```python
from build123d import *

# Parameters (mm, degrees)
SKETCH2_R                 = 3.2
FRONT_MOUNTING_DEPTH      = 10.65
FRONT_MOUNTING_DEPTH_BACK = 10.65


with BuildPart() as part:
    # Sketch1 → Body (revolve)
    with BuildSketch(Plane(origin=(0, 0, 0), x_dir=(0, 0, -1), z_dir=(1, 0, 0))):
        Polygon((51.45, 9.65), (50.2, 8.4), (48.95, 9.65), (-31, 9.65), (-31, 0), (67.4, 0), (67.4, 9.65), (57.7, 9.65), align=None)
    revolve(axis=Axis((0, 0, -67.4), (0, 0, 1)))

    # Sketch2 → Front-Mounting (cut, two sides)
    with BuildSketch(Plane(origin=(0, 0, 0), x_dir=(0, 0, -1), z_dir=(1, 0, 0))) as front_mounting_sk:
        with Locations((57.7, 0)):
            Circle(SKETCH2_R)
    extrude(amount=FRONT_MOUNTING_DEPTH, mode=Mode.SUBTRACT)
    extrude(front_mounting_sk.sketch, amount=-FRONT_MOUNTING_DEPTH_BACK, mode=Mode.SUBTRACT)


solid = part.part
```
The listing builds one solid part. Answer for the finished solid, in the listing's coordinates (mm). A direction names the side the tool comes from. Round coordinates to 2 decimals unless told otherwise and drop trailing zeros. Loops run counter-clockwise (first coordinate to the right, second up) from the corner with the lowest first, then second, coordinate; pieces in that order, holes last.
1) A cutting plane is placed at C-C on z = -53. Determine the outline of the cut face in (x, y), plus the area to 3 significant figures.
Outcome:
outline: circle Ø19.3 at (0, 0)
area: 293 mm2
2) Given P1, Ø1.5, axis at x = 5, z = -3, coming from the -Y side; P2, Ø6, axis at x = -6, z = -6.5, coming from the +Y side; P3, Ø6, axis at y = 0, z = -57.7, coming from the -X side; P4, Ø6, axis at y = -4, z = -50.5, coming from the +X side, each flat-ended and moving along its own axis, determine where each tip first touches the part or whether it passes through.
Outcome:
P1: stops at y = -8.66
P2: stops at y = 9.17
P3: passes through
P4: stops at x = 9.58
3) For a pull along Z with two mould halves and no side action, classify faces 3 (the face through (-2.899, 9.204, -8.415)), 4 (the face through (0, 0, 31)), 5 (the face through (0.1, 0.1, -54.5)) as released by +Z, released by -Z, zero draft, split by the parting line, or undercut.
Outcome:
face 3: zero draft
face 4: released by +Z
face 5: undercut
4) For faces 1 (the face through (0, 0, -67.4)), 2 (the face through (-7, 5, -50)), determine the directions among +Z, -Z, +X, -X, +Y, -Y from which every point of the face is accessible in a straight line to the end or side of a thin tool.
Outcome:
face 1: -Z, +X, -X, +Y, -Y
face 2: none
5) Consider line 1 (Z direction, x = -1, y = 0); line 2 (Z direction, x = -0.5, y = 0.75); line 3 (Y direction, x = 5.75, z = -57.5). Determine where each line is inside the solid, lowest interval first.
Outcome:
line 1: z = -67.4 to -60.9, -54.5 to 31
line 2: z = -67.4 to -60.81, -54.59 to 31
line 3: y = -7.75 to -3.19, 3.19 to 7.75
6) A cutting plane is placed at A-A on x = 0. Determine the outline of the cut face in (y, z).
Outcome:
outline: (-9.65, -67.4) - (9.65, -67.4) - (9.65, -51.45) - (8.4, -50.2) - (9.65, -48.95) - (9.65, 31) - (-9.65, 31) - (-9.65, -48.95) - (-8.4, -50.2) - (-9.65, -51.45) - close; hole circle Ø6.4 at (0, -57.7)
7) A cutting plane is placed at B-B on y = 0. Determine the outline of the cut face in (x, z).
Outcome:
outline: (-9.65, -67.4) - (9.65, -67.4) - (9.65, -60.9) - (-9.65, -60.9) - close; (-9.65, -54.5) - (9.65, -54.5) - (9.65, -51.45) - (8.4, -50.2) - (9.65, -48.95) - (9.65, 31) - (-9.65, 31) - (-9.65, -48.95) - (-8.4, -50.2) - (-9.65, -51.45) - close
